Geometry: final body of the model. Coordinates: model frame, mm. A direction names the side the tool comes from. Give positions to 0.01 mm unless a question says otherwise; leave off trailing zeros. Use one line per item in the form item = value.
```python
from build123d import *

# Parameters (mm, degrees)
SKETCH_1_W             = 23.5
SKETCH_1_H             = 12
EXTRUDE_1_DEPTH        = 571
HOLE_WIZARD_M6_1_D     = 5
HOLE_WIZARD_M6_1_DEPTH = 15
HOLE_WIZARD_M6_1_TIP   = 1.502151548
HOLE_WIZARD_M6_2_D     = 5
HOLE_WIZARD_M6_2_DEPTH = 15
HOLE_WIZARD_M6_2_TIP   = 1.502151548
HOLE_WIZARD_M6_3_D     = 5
HOLE_WIZARD_M6_3_DEPTH = 15
HOLE_WIZARD_M6_3_TIP   = 1.502151548
HOLE_WIZARD_M4_1_D     = 3.3
HOLE_WIZARD_M4_1_DEPTH = 10.1
HOLE_WIZARD_M4_1_TIP   = 0.991420021


with BuildPart() as part:
    # 草图1 → 凸台-拉伸1 (new, symmetric)
    with BuildSketch(Plane(origin=(0, 0, 0), x_dir=(0, 0, -1), z_dir=(1, 0, 0))):
        with BuildLine():
            Line((-14, 15), (-11.5, 15))
            Line((-11.5, 15), (-11.5, 13.5))
            Line((-11.5, 13.5), (-11.4, 13.5))
            ThreePointArc((-11.4, 13.5), (-11.117157288, 13.382842712), (-11, 13.1))
            Line((-11, 13.1), (-11, 12))
            Line((-11, 12), (-9.5, 12))
            Line((-9.5, 12), (-9.5, 15))
            Line((-9.5, 15), (-8, 15))
            Line((-8, 15), (-8, 12.5))
            Line((-8, 12.5), (-5, 12.5))
            Line((-5, 12.5), (-5, 15))
            Line((-5, 15), (5, 15))
            Line((5, 15), (5, 12.5))
            Line((5, 12.5), (8, 12.5))
            Line((8, 12.5), (8, 15))
            Line((8, 15), (9.5, 15))
            Line((9.5, 15), (9.5, 12))
            Line((9.5, 12), (11, 12))
            Line((11, 12), (11, 13.1))
            ThreePointArc((11, 13.1), (11.117157288, 13.382842712), (11.4, 13.5))
            Line((11.4, 13.5), (11.5, 13.5))
            Line((11.5, 13.5), (11.5, 15))
            Line((11.5, 15), (14, 15))
            ThreePointArc((14, 15), (14.707106781, 14.707106781), (15, 14))
            Line((15, 14), (15, 8))
            Line((15, 8), (12.5, 8))
            Line((12.5, 8), (12.5, 5))
            Line((12.5, 5), (15, 5))
            Line((15, 5), (15, -5))
            Line((15, -5), (12.5, -5))
            Line((12.5, -5), (12.5, -8))
            Line((12.5, -8), (15, -8))
            Line((15, -8), (15, -14))
            ThreePointArc((15, -14), (14.707106781, -14.707106781), (14, -15))
            Line((14, -15), (11.5, -15))
            Line((11.5, -15), (11.5, -13.5))
            Line((11.5, -13.5), (11.4, -13.5))
            ThreePointArc((11.4, -13.5), (11.117157288, -13.382842712), (11, -13.1))
            Line((11, -13.1), (11, -12))
            Line((11, -12), (9.5, -12))
            Line((9.5, -12), (9.5, -15))
            Line((9.5, -15), (8, -15))
            Line((8, -15), (8, -12.5))
            Line((8, -12.5), (5, -12.5))
            Line((5, -12.5), (5, -15))
            Line((5, -15), (-5, -15))
            Line((-5, -15), (-5, -12.5))
            Line((-5, -12.5), (-8, -12.5))
            Line((-8, -12.5), (-8, -15))
            Line((-8, -15), (-9.5, -15))
            Line((-9.5, -15), (-9.5, -12))
            Line((-9.5, -12), (-11, -12))
            Line((-11, -12), (-11, -13.1))
            ThreePointArc((-11, -13.1), (-11.117157288, -13.382842712), (-11.4, -13.5))
            Line((-11.4, -13.5), (-11.5, -13.5))
            Line((-11.5, -13.5), (-11.5, -15))
            Line((-11.5, -15), (-14, -15))
            ThreePointArc((-14, -15), (-14.707106781, -14.707106781), (-15, -14))
            Line((-15, -14), (-15, 14))
            ThreePointArc((-15, 14), (-14.707106781, 14.707106781), (-14, 15))
        make_face()
        with BuildLine():
            Line((12, -10.5), (12, -8.5))
            ThreePointArc((12, -8.5), (11.853553391, -8.146446609), (11.5, -8))
            Line((11.5, -8), (-11.5, -8))
            ThreePointArc((-11.5, -8), (-11.853553391, -8.146446609), (-12, -8.5))
            Line((-12, -8.5), (-12, -10.5))
            ThreePointArc((-12, -10.5), (-11.853553391, -10.853553391), (-11.5, -11))
            Line((-11.5, -11), (11.5, -11))
            ThreePointArc((11.5, -11), (11.853553391, -10.853553391), (12, -10.5))
        make_face(mode=Mode.SUBTRACT)
        with BuildLine():
            Line((-11.5, 11), (11.5, 11))
            ThreePointArc((11.5, 11), (11.853553391, 10.853553391), (12, 10.5))
            Line((12, 10.5), (12, 8.5))
            ThreePointArc((12, 8.5), (11.853553391, 8.146446609), (11.5, 8))
            Line((11.5, 8), (-11.5, 8))
            ThreePointArc((-11.5, 8), (-11.853553391, 8.146446609), (-12, 8.5))
            Line((-12, 8.5), (-12, 10.5))
            ThreePointArc((-12, 10.5), (-11.853553391, 10.853553391), (-11.5, 11))
        make_face(mode=Mode.SUBTRACT)
        Rectangle(SKETCH_1_W, SKETCH_1_H, mode=Mode.SUBTRACT)
    extrude(amount=EXTRUDE_1_DEPTH, both=True)

    # M6 螺纹孔1
    with Locations(Plane(origin=(0, 15, 0), x_dir=(-1, 0, 0), z_dir=(0, 1, 0))):
        with Locations((551, 0), (536, 0), (236, 0), (221, 0), (151, 0), (136, 0), (-536, 0), (-551, 0)):
            Hole(HOLE_WIZARD_M6_1_D / 2, depth=HOLE_WIZARD_M6_1_DEPTH)
            with Locations((0, 0, -(HOLE_WIZARD_M6_1_DEPTH + HOLE_WIZARD_M6_1_TIP / 2))):  # 118° drill point
                Cone(0, HOLE_WIZARD_M6_1_D / 2, HOLE_WIZARD_M6_1_TIP, mode=Mode.SUBTRACT)

    # M6 螺纹孔2
    with Locations(Plane.XZ.offset(15)):
        with Locations((-551, 0), (-536, 0), (536, 0), (551, 0)):
            Hole(HOLE_WIZARD_M6_2_D / 2, depth=HOLE_WIZARD_M6_2_DEPTH)
            with Locations((0, 0, -(HOLE_WIZARD_M6_2_DEPTH + HOLE_WIZARD_M6_2_TIP / 2))):  # 118° drill point
                Cone(0, HOLE_WIZARD_M6_2_D / 2, HOLE_WIZARD_M6_2_TIP, mode=Mode.SUBTRACT)

    # M6 螺纹孔3
    with Locations(Plane(origin=(0, 0, -15), x_dir=(-1, 0, 0), z_dir=(0, 0, -1))):
        with Locations((293.5, 0), (218.5, 0)):
            Hole(HOLE_WIZARD_M6_3_D / 2, depth=HOLE_WIZARD_M6_3_DEPTH)
            with Locations((0, 0, -(HOLE_WIZARD_M6_3_DEPTH + HOLE_WIZARD_M6_3_TIP / 2))):  # 118° drill point
                Cone(0, HOLE_WIZARD_M6_3_D / 2, HOLE_WIZARD_M6_3_TIP, mode=Mode.SUBTRACT)

    # M4 螺纹孔1
    with Locations(Plane.XZ.offset(15)):
        with Locations((-326, 0), (-131, 0), (64, 0), (259, 0), (454, 0)):
            Hole(HOLE_WIZARD_M4_1_D / 2, depth=HOLE_WIZARD_M4_1_DEPTH)
            with Locations((0, 0, -(HOLE_WIZARD_M4_1_DEPTH + HOLE_WIZARD_M4_1_TIP / 2))):  # 118° drill point
                Cone(0, HOLE_WIZARD_M4_1_D / 2, HOLE_WIZARD_M4_1_TIP, mode=Mode.SUBTRACT)


solid = part.part
```
(1) Cut plane A-A (x = 199). Give the number of separate pieces and of enclosed holes in the cut face, plus the area to 3 significant figures.
Solution:
separate_pieces = 1
enclosed_holes = 3
area = 407 mm2
(2) Pin query (flat end, axial travel): P1, Ø1.5, axis at x = 69, y = 7, coming from the -Z side. Return the tip coordinate at first contact, or that it passes through.
Solution:
P1 = -12.5
(3) Material intervals for L1, parallel to Y at x = -465.5, z = 1; L2, parallel to Y at x = -494, z = -14; L3, parallel to Z at x = -536, y = 12.25, sorted ascending. Write a range as from..to.
Solution:
L1 = -15..-11, -8..-6, 6..8, 11..15
L2 = -15..-8, -5..5, 8..15
L3 = -15..-11, -9.5..-2.5, 2.5..9.5, 11..15
(4) Access query for faces 4 (the face through (571, 7, 0)), 5 (the face through (8, 8, 0)). Directions: +Z, -Z, +X, -X, +Y, -Y. A direction counts if a zero-diameter tool reaches every point of the face in a straight line with its end or side. Return the directions, or none.
Solution:
face_4 = +Z, -Z, +X, +Y, -Y
face_5 = +X, -X
(5) Pull-direction query (Z, two-part tool) for faces 1 (the face through (8, 6, 0)), 2 (the face through (8, 0, 15)), 3 (the face through (-571, 7, 0)); classes: released by +Z, released by -Z, zero draft, split by the parting line, or undercut.
Solution:
face_1 = undercut
face_2 = released by +Z
face_3 = zero draft
